from build123d import *

# Parameters (mm, degrees)
F0_R     = 12.7
F1_DEPTH = 3.175


with BuildPart() as f1:
    # F0 (on Front) → F1 (new body)
    with BuildSketch(Plane.XZ):
        with Locations((0, -0.918301)):
            Circle(F0_R)
        Polygon((-10.76945, -2.039835), (-10.76945, 1.764737), (-1.902286, 1.764737), (-1.902286, 10.01233), (1.902286, 10.01233), (1.902286, 1.764737), (10.76945, 1.764737), (10.76945, -2.039835), (1.902286, -2.039835), (1.902286, -11.573113), (-1.902286, -11.573113), (-1.902286, -2.039835), align=None, mode=Mode.SUBTRACT)
    extrude(amount=F1_DEPTH)


solid = f1.part
Can you work these out from the model? Positions are in its coordinate system, mm. A direction names the side the tool comes from. Coordinates: 2 decimals unless noted, no trailing zeros. Loops run counter-clockwise (first coordinate to the right, second up) from the corner with the lowest first, then second, coordinate; pieces in that order, holes last. Notation, with made-up numbers: M -29,69 L -16,69 A18 ccw -16,87 Z; hole C 27,24 d7. An arc over 180 degrees is marked long. Return JSON: item names as keys, results as strings. Group by question number.
Item 1: Imagine slicing it at B-B (z = 4.25). Please give me the cut outline in (x, y) (3 decimals), and give its area (3 significant figures).
Item 2: Imagine slicing it at A-A (x = 0). Please give me the cut outline in (y, z) (3 decimals), and give its area (3 significant figures).
Item 3: I'm going to push flat-ended pins straight in: pin 1 Ø1 at (y, z) = (-2, -6.5) entering from +X; pin 2 Ø1 at (x, y) = (8, -1) entering from +Z; pin 3 Ø1.6 at (x, y) = (4.5, -1) entering from -Z. Where does each tip first touch, or does it pass through?
Item 4: If I drill on L1, parallel to Z at x = -9.5, y = -0.05; L2, parallel to X at y = -1.15, z = -3; L3, parallel to X at y = -1.3, z = 2.75, over which ranges is the centre line in solid material (lowest first)? Write a range as from..to.
Item 5: Thinking about a two-plate mould opening in X: for faces 1 (the flat face through (3, -3.175, -4)), 2 (the flat face through (0, -2, 10.012)), 3 (the flat face through (0, -2, -11.573)), 4 (the cylindrical face through (-2.753, -1.565, -13.316)), which applies, released by +X, released by -X, zero draft, split by the parting line, or undercut?
Item 6: On a 3-axis mill with a long thin cutter (end or side, diameter ignored), from which of +Z, -Z, +X, -X, +Y, -Y can I reach the whole of each face in a straight line? I mean faces 5 (the flat face through (1.902, -2, 6)), 6 (the flat face through (3, 0, -4)). Say none if no direction works.
Item 7: Imagine slicing it at C-C (y = -1.65). Please give me the cut outline in (x, z).
Verdict:
{
 "1": {"outline": "M -11.601,-3.175 L -1.902,-3.175 L -1.902,0 L -11.601,0 Z; M 1.902,-3.175 L 11.601,-3.175 L 11.601,0 L 1.902,0 Z", "area": "61.6 mm^2"},
 "2": {"outline": "M -3.175,-13.618 L 0,-13.618 L 0,-11.573 L -3.175,-11.573 Z; M -3.175,10.012 L 0,10.012 L 0,11.782 L -3.175,11.782 Z", "area": "12.1 mm^2"},
 "3": {"pin 1": "stops at x = 11.64", "pin 2": "stops at z = 9.33", "pin 3": "stops at z = -13.07"},
 "4": {"L1": "z = -9.35..-2.04, 1.76..7.51", "L2": "x = -12.53..-1.9, 1.9..12.53", "L3": "x = -12.16..-1.9, 1.9..12.16"},
 "5": {"face 1": "zero draft", "face 2": "undercut", "face 3": "undercut", "face 4": "split by the parting line"},
 "6": {"face 5": "+Y, -Y", "face 6": "+Z, -Z, +X, -X, +Y"},
 "7": {"outline": "C 0,-0.92 d25.4; hole M -10.77,-2.04 L -1.9,-2.04 L -1.9,-11.57 L 1.9,-11.57 L 1.9,-2.04 L 10.77,-2.04 L 10.77,1.76 L 1.9,1.76 L 1.9,10.01 L -1.9,10.01 L -1.9,1.76 L -10.77,1.76 Z"}
}
